```python
from build123d import *

# Parameters (mm, degrees)
F0_R     = 4.6
F0_R_2   = 8.05
F1_DEPTH = 10
F0_R_3   = 2.5
F2_DEPTH = 3


# Not quite as in the source:
# - ends of sketch curves that miss each other by under 0.0002 mm in the source are joined


with BuildPart() as f1:
    # F0 (on Top) → F1 (new body)
    with BuildSketch(Plane.XY):
        with BuildLine():
            ThreePointArc((-30, -34.104246), (-29.5606601718, -35.1649061718), (-28.5, -35.604246))
            Line((-28.5, -35.604246), (28.5, -35.604246))
            ThreePointArc((28.5, -35.604246), (29.5606601718, -35.1649061718), (30, -34.104246))
            Line((30, -34.104246), (30, -14.645125))
            ThreePointArc((30, -14.645125), (30.1141807012, -14.0710998515), (30.4393398282, -13.5844648282))
            Line((30.4393398282, -13.5844648282), (37.314025, -6.70978))
            ThreePointArc((37.314025, -6.70978), (38.778491, -3.174246), (37.3140249059, 0.3612879059))
            Line((37.3140249059, 0.3612879059), (3.535534, 34.139779))
            ThreePointArc((3.535534, 34.139779), (0, 35.604245), (-3.5355339059, 34.1397789059))
            Line((-3.5355339059, 34.1397789059), (-37.314025, 0.361288))
            ThreePointArc((-37.314025, 0.361288), (-38.778491, -3.174246), (-37.3140249059, -6.7097799059))
            Line((-37.3140249059, -6.7097799059), (-30.43934, -13.584465))
            ThreePointArc((-30.43934, -13.584465), (-30.1141807012, -14.0710998515), (-30, -14.645125))
            Line((-30, -14.645125), (-30, -34.104246))
        make_face()
        with BuildLine():
            ThreePointArc((-24.6, -20.174246), (-20, -15.574246), (-15.4, -20.174246))
            Line((-15.4, -20.174246), (-15.4, -26.974246))
            ThreePointArc((-15.4, -26.974246), (-20, -31.574246), (-24.6, -26.974246))
            Line((-24.6, -26.974246), (-24.6, -20.174246))
        make_face(mode=Mode.SUBTRACT)
        with Locations((-33.333, -3.174246)):
            Circle(F0_R, mode=Mode.SUBTRACT)
        with BuildLine():
            ThreePointArc((4.6, -26.974246), (0, -31.574246), (-4.6, -26.974246))
            Line((-4.6, -26.974246), (-4.6, -20.174246))
            ThreePointArc((-4.6, -20.174246), (0, -15.574246), (4.6, -20.174246))
            Line((4.6, -20.174246), (4.6, -26.974246))
        make_face(mode=Mode.SUBTRACT)
        with BuildLine():
            ThreePointArc((24.6, -26.974246), (20, -31.574246), (15.4, -26.974246))
            Line((15.4, -26.974246), (15.4, -20.174246))
            ThreePointArc((15.4, -20.174246), (20, -15.574246), (24.6, -20.174246))
            Line((24.6, -20.174246), (24.6, -26.974246))
        make_face(mode=Mode.SUBTRACT)
        with Locations((0, -3.174246)):
            Circle(F0_R_2, mode=Mode.SUBTRACT)
        with Locations((33.333, -3.174246)):
            Circle(F0_R, mode=Mode.SUBTRACT)
        with Locations((0, 30.158782)):
            Circle(F0_R, mode=Mode.SUBTRACT)
    extrude(amount=F1_DEPTH)

    # F0 (on Top) → F2 (join)
    with BuildSketch(Plane.XY):
        with Locations((-33.333, -3.174246)):
            Circle(F0_R)
        with Locations((-33.333, -3.174246)):
            Circle(F0_R_3, mode=Mode.SUBTRACT)
        with BuildLine():
            Line((-15.4, -26.974246), (-15.4, -20.174246))
            ThreePointArc((-15.4, -20.174246), (-20, -15.574246), (-24.6, -20.174246))
            Line((-24.6, -20.174246), (-24.6, -26.974246))
            ThreePointArc((-24.6, -26.974246), (-20, -31.574246), (-15.4, -26.974246))
        make_face()
        with BuildLine():
            ThreePointArc((-17.5, -26.974246), (-20, -29.474246), (-22.5, -26.974246))
            Line((-22.5, -26.974246), (-22.5, -20.174246))
            ThreePointArc((-22.5, -20.174246), (-20, -17.674246), (-17.5, -20.174246))
            Line((-17.5, -20.174246), (-17.5, -26.974246))
        make_face(mode=Mode.SUBTRACT)
        with BuildLine():
            Line((-4.6, -20.174246), (-4.6, -26.974246))
            ThreePointArc((-4.6, -26.974246), (0, -31.574246), (4.6, -26.974246))
            Line((4.6, -26.974246), (4.6, -20.174246))
            ThreePointArc((4.6, -20.174246), (0, -15.574246), (-4.6, -20.174246))
        make_face()
        with BuildLine():
            ThreePointArc((2.5, -26.974246), (0, -29.474246), (-2.5, -26.974246))
            Line((-2.5, -26.974246), (-2.5, -20.174246))
            ThreePointArc((-2.5, -20.174246), (0, -17.674246), (2.5, -20.174246))
            Line((2.5, -20.174246), (2.5, -26.974246))
        make_face(mode=Mode.SUBTRACT)
        with BuildLine():
            Line((15.4, -20.174246), (15.4, -26.974246))
            ThreePointArc((15.4, -26.974246), (20, -31.574246), (24.6, -26.974246))
            Line((24.6, -26.974246), (24.6, -20.174246))
            ThreePointArc((24.6, -20.174246), (20, -15.574246), (15.4, -20.174246))
        make_face()
        with BuildLine():
            ThreePointArc((22.5, -26.974246), (20, -29.474246), (17.5, -26.974246))
            Line((17.5, -26.974246), (17.5, -20.174246))
            ThreePointArc((17.5, -20.174246), (20, -17.674246), (22.5, -20.174246))
            Line((22.5, -20.174246), (22.5, -26.974246))
        make_face(mode=Mode.SUBTRACT)
        with Locations((33.333, -3.174246)):
            Circle(F0_R)
        with Locations((33.333, -3.174246)):
            Circle(F0_R_3, mode=Mode.SUBTRACT)
        with Locations((0, 30.158782)):
            Circle(F0_R)
        with Locations((0, 30.158782)):
            Circle(F0_R_3, mode=Mode.SUBTRACT)
    extrude(amount=F2_DEPTH)


solid = f1.part
```
Design review of the part built by this model. Coordinates are the model's own, in mm. A direction names the side the tool comes from. Coordinates: 2 decimals unless noted, no trailing zeros. Order: outer loops, then holes, each group sorted by start corner. A loop starts at its lowest first (then second) coordinate and runs counter-clockwise, first axis right, second up.
1) For faces 4 (the flat face through (15.4, -24, 6)), 5 (the cylindrical face through (-19.945, -29.474, 1.479)), 6 (the cylindrical face through (-38.78, -3.12, 4.93)), list the 3-axis set-ups (+Z, -Z, +X, -X, +Y, -Y) from which the entire face can be reached by the end or side of a thin tool; tool diameter is ignored.
2) Wall thickness on line 1 along Y through (x, z) = (0, 4); line 2 along X through (y, z) = (-3, 9.5); line 3 along Y through (x, z) = (-3, 3.25): over which ranges is each line inside the solid? List them lowest first.
3) Take a section at C-C, the plane x = 20. Give the boundary of the cut face in (y, z), and give its area (3 significant figures).
4) Take a section at D-D, the plane y = 9.5. Give the boundary of the cut face in (x, z).
5) Mouldability with a two-part tool opening along X and no side actions: class faces 1 (the flat face through (-9, -7, 10)), 2 (the cylindrical face through (0.101, -31.573, 6.451)), 3 (the flat face through (-30, -24, 5)) as +X half, -X half, draft (parallel to the pull), parting line (faces both ways), or undercut.
6) Take a section at B-B, the plane z = 8.25. State how many separate pieces and enclosed holes the cut face has, and give its area (3 significant figures).
7) Take a section at A-A, the plane x = 0. Give the boundary of the cut face in (y, z).
8) Clearance check with flat-ended pins moving along their axes: pin 1 (1.5 mm diameter, centred on y = -24, z = 1, fed in from -X); pin 2 (3 mm diameter, centred on y = -24, z = 4.5, fed in from +X); pin 3 (5 mm diameter, centred on y = 24, z = 7, fed in from +X); pin 4 (3 mm diameter, centred on x = 33.33, y = -3.17, fed in from -Z). State where each tip first meets the part, or that it passes through.
Returned:
1. face 4: +Z
1. face 5: +Z, -Z
1. face 6: +Z, -Z, -X
2. line 1: y = -35.6 to -31.57, -15.57 to -11.22, 4.88 to 25.56, 34.76 to 35.6
2. line 2: x = -38.78 to -37.93, -28.74 to -8.05, 8.05 to 28.74, 37.93 to 38.78
2. line 3: y = -35.6 to -30.46, -16.69 to -10.64, 4.3 to 26.67, 33.65 to 34.6
3. outline: (-35.6, 0) - (-29.47, 0) - (-29.47, 3) - (-31.57, 3) - (-31.57, 10) - (-35.6, 10) - close; (-17.67, 0) - (17.68, 0) - (17.68, 10) - (-15.57, 10) - (-15.57, 3) - (-17.67, 3) - close
3. area: 385 mm2
4. outline: (-28.18, 0) - (28.18, 0) - (28.18, 10) - (-28.18, 10) - close
5. face 1: draft
5. face 2: undercut
5. face 3: -X half
6. separate pieces: 1
6. enclosed holes: 7
6. area: 2,930 mm2
7. outline: (-35.6, 0) - (-29.47, 0) - (-29.47, 3) - (-31.57, 3) - (-31.57, 10) - (-35.6, 10) - close; (-17.67, 0) - (-11.22, 0) - (-11.22, 10) - (-15.57, 10) - (-15.57, 3) - (-17.67, 3) - close; (4.88, 0) - (27.66, 0) - (27.66, 3) - (25.56, 3) - (25.56, 10) - (4.88, 10) - close; (32.66, 0) - (35.6, 0) - (35.6, 10) - (34.76, 10) - (34.76, 3) - (32.66, 3) - close
8. pin 1: stops at x = -30
8. pin 2: stops at x = 30
8. pin 3: stops at x = 16.18
8. pin 4: passes through
